Source: CAD feature listing. Evaluate the final solid. Frame: model axes, mm. Face numbers are marked on the shaded views. A direction names the side the tool comes from. Round coordinates to 2 decimals unless told otherwise and drop trailing zeros. Loops run counter-clockwise (first coordinate to the right, second up) from the corner with the lowest first, then second, coordinate; pieces in that order, holes last.
(1) Material intervals for probe 1 along X at (y, z) = (10.75, -21); probe 2 along Z at (x, y) = (-6.75, 6); probe 3 along Y at (x, z) = (-3, -19), sorted ascending.
(2) Section C-C, the plane x = -3.5. Return the cut outline in (y, z), plus the area to 3 significant figures.
(3) Set-up query: the marked faces 1, 2, 3 and 4. Return all of +Z, -Z, +X, -X, +Y, -Y with unobstructed straight access to the full face (end or side cutting, diameter ignored); none if empty.
(4) Section D-D, the plane z = 20. Return the cut outline in (x, y), plus the area to 3 significant figures.
(5) Section A-A, the plane y = 1.5. Return the cut outline in (x, z), plus the area to 3 significant figures.
(6) First-contact query: pin 1 Ø0.8 at (y, z) = (2, 10) entering from -X; pin 2 Ø8 at (y, z) = (5, 13.5) entering from +X; pin 3 Ø2 at (y, z) = (1.5, 9) entering from +X. Flat tips, straight axial feed; report the tip coordinate or a pass-through.
(7) Section B-B, the plane z = 1.5. Return the cut outline in (x, y).
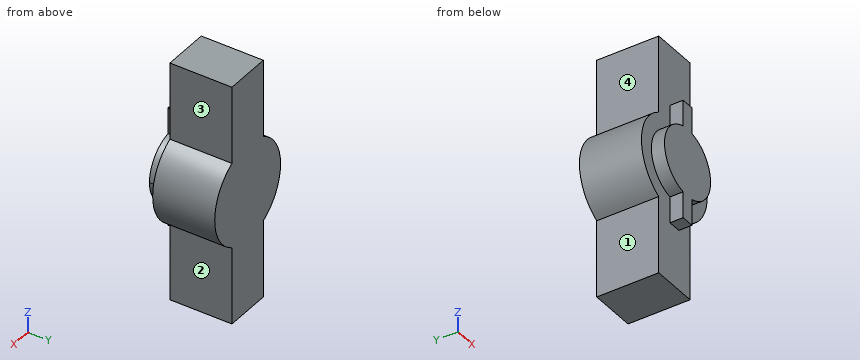
```python
from build123d import *

# Parameters (mm, degrees)
BOSS_EXTRUDE1_DEPTH = 2.54
BOSS_EXTRUDE2_DEPTH = 12


with BuildPart() as part:
    # Sketch1 → Boss-Extrude1 (new body)
    with BuildSketch(Plane(origin=(0, 0, 0), x_dir=(1, 0, 0), z_dir=(0, 1, 0))):
        with BuildLine():
            ThreePointArc((1.27, -6.480734218), (0, -6.604), (-1.27, -6.480734218))
            Line((-1.27, -6.480734218), (-1.27, -11.560734218))
            Line((-1.27, -11.560734218), (1.27, -11.560734218))
            Line((1.27, -11.560734218), (1.27, -6.480734218))
        make_face()
        with BuildLine():
            ThreePointArc((1.27, 6.480734218), (0, 6.604), (-1.27, 6.480734218))
            ThreePointArc((-1.27, 6.480734218), (-6.604, 0), (-1.27, -6.480734218))
            ThreePointArc((-1.27, -6.480734218), (0, -6.604), (1.27, -6.480734218))
            ThreePointArc((1.27, -6.480734218), (5.099014415, -4.196768757), (6.604, 0))
            ThreePointArc((6.604, 0), (5.099014415, 4.196768757), (1.27, 6.480734218))
        make_face()
        with BuildLine():
            Line((-1.27, 11.560734218), (-1.27, 6.480734218))
            ThreePointArc((-1.27, 6.480734218), (0, 6.604), (1.27, 6.480734218))
            Line((1.27, 6.480734218), (1.27, 11.560734218))
            Line((1.27, 11.560734218), (-1.27, 11.560734218))
        make_face()
    extrude(amount=BOSS_EXTRUDE1_DEPTH)

    # Sketch2 → Boss-Extrude2 (add)
    with BuildSketch(Plane(origin=(0, 2.54, 0), x_dir=(1, 0, 0), z_dir=(0, 1, 0))):
        with BuildLine():
            Line((-4.5, 8.309783391), (-4.5, 23.309783391))
            Line((-4.5, 23.309783391), (4.5, 23.309783391))
            Line((4.5, 23.309783391), (4.5, 8.309783391))
            ThreePointArc((4.5, 8.309783391), (9.45, 0), (4.5, -8.309783391))
            Line((4.5, -8.309783391), (4.5, -23.309783391))
            Line((4.5, -23.309783391), (-4.5, -23.309783391))
            Line((-4.5, -23.309783391), (-4.5, -8.309783391))
            ThreePointArc((-4.5, -8.309783391), (-9.45, 0), (-4.5, 8.309783391))
        make_face()
    extrude(amount=BOSS_EXTRUDE2_DEPTH)


solid = part.part
```
Output values:
1. probe 1: x = -4.5 to 4.5
1. probe 2: z = -6.61 to 6.61
1. probe 3: y = 2.54 to 14.54
2. outline: (0, -5.6) - (2.54, -5.6) - (2.54, -23.31) - (14.54, -23.31) - (14.54, 23.31) - (2.54, 23.31) - (2.54, 5.6) - (0, 5.6) - close
2. area: 588 mm2
3. face 1: -Z, -X, +Y, -Y
3. face 2: -Z, +X, +Y, -Y
3. face 3: +Z, +X, +Y, -Y
3. face 4: +Z, -X, +Y, -Y
4. outline: (-4.5, 2.54) - (4.5, 2.54) - (4.5, 14.54) - (-4.5, 14.54) - close
4. area: 108 mm2
5. outline: (-1.27, -11.56) - (1.27, -11.56) - (1.27, -6.48) arc R6.6 ccw to (1.27, 6.48) - (1.27, 11.56) - (-1.27, 11.56) - (-1.27, 6.48) arc R6.6 ccw to (-1.27, -6.48) - close
5. area: 162 mm2
6. pin 1: stops at x = -1.27
6. pin 2: stops at x = 4.5
6. pin 3: stops at x = 1.27
7. outline: (-9.33, 2.54) - (-6.43, 2.54) - (-6.43, 0) - (6.43, 0) - (6.43, 2.54) - (9.33, 2.54) - (9.33, 14.54) - (-9.33, 14.54) - close
